Read the model definition and answer for the solid it produces. Units are mm, in the model's axes. A direction names the side the tool comes from. Coordinates: 2 decimals unless noted, no trailing zeros. Write each loop counter-clockwise with the first axis right and the second up, starting at its lowest first coordinate (ties: lowest second). Pieces come first, ordered by that corner, then holes. Notation, with made-up numbers: (34, 58.25) - (49, 58.25) arc R31 cw to (49, 82.25) - close; hole circle Ø10 at (47.25, -39). An arc over 180 degrees is marked (long way). Return JSON: item names as keys, results as strings.
```python
from build123d import *

# Parameters (mm, degrees)
F1_DEPTH = 500
F2_DEPTH = 311.15


with BuildPart() as f1:
    # F0 (on Front) → F1 (new body)
    with BuildSketch(Plane.XZ):
        with BuildLine():
            ThreePointArc((-155.575, 0), (0, -155.575), (155.575, 0))
            ThreePointArc((155.575, 0), (0, 155.575), (-155.575, 0))
        make_face()
    extrude(amount=F1_DEPTH)

    # F0 (on Front) → F2 (join)
    with BuildSketch(Plane.XZ):
        with BuildLine():
            ThreePointArc((-155.575, 0), (0, -155.575), (155.575, 0))
            ThreePointArc((155.575, 0), (0, 155.575), (-155.575, 0))
        make_face()
        with BuildLine():
            Line((155.575, -200), (155.575, 0))
            ThreePointArc((155.575, 0), (0, -155.575), (-155.575, 0))
            Line((-155.575, 0), (-155.575, -200))
            Line((-155.575, -200), (155.575, -200))
        make_face()
    extrude(amount=-F2_DEPTH)


solid = f1.part
```
(1) Straight lines are drawn through the part: line 1 (Z direction, x = -5, y = -41.5); line 2 (Z direction, x = 71.5, y = -146); line 3 (X direction, y = -204, z = 140.5). For each, find the intervals that lie inside material, in ascending order. Write a range as from..to.
Answer:
{"line 1": "-155.49..155.49", "line 2": "-138.17..138.17", "line 3": "-66.81..66.81"}
(2) Flat-ended cylindrical pins translate along their axes: P1, Ø1.5, axis at y = -179.5, z = 79.5, coming from the +X side; P2, Ø1.5, axis at y = -87, z = -89, coming from the +X side; P3, Ø10, axis at y = -241, z = 113.5, coming from the -X side. Find the tip coordinate at first contact, or state that the pin passes through.
Answer:
{"P1": "x = 134.17", "P2": "x = 128.12", "P3": "x = -111.5"}
(3) A cutting plane is placed at D-D (x = 0). Determine the outline of the cut face in (y, z) (3 decimals), and give its area (3 significant figures).
Answer:
{"outline": "(-500, -155.575) - (0, -155.575) - (0, -200) - (311.15, -200) - (311.15, 155.575) - (-500, 155.575) - close", "area": "266,000 mm²"}
(4) Which of the six approach directions +Z, -Z, +X, -X, +Y, -Y give full straight-line access (tool end or side, diameter ignored) to faces 1 (the face through (-2, 0, -165)), 2 (the face through (155.575, 153, -101))?
Answer:
{"face 1": "-Z, -Y", "face 2": "+Z, -Z, +X, +Y, -Y"}
(5) A cutting plane is placed at C-C (y = 184). Determine the outline of the cut face in (x, z) (3 decimals).
Answer:
{"outline": "(-155.575, -200) - (155.575, -200) - (155.575, 0) arc R155.575 ccw to (-155.575, 0) - close"}
(6) A cutting plane is placed at B-B (x = -124). Determine the outline of the cut face in (y, z), and give its area (3 significant figures).
Answer:
{"outline": "(-500, -93.96) - (0, -93.96) - (0, -200) - (311.15, -200) - (311.15, 93.96) - (-500, 93.96) - close", "area": "185,000 mm²"}
(7) A cutting plane is placed at A-A (z = -45.5). Determine the outline of the cut face in (x, y) (3 decimals).
Answer:
{"outline": "(-155.575, 0) - (-148.773, 0) - (-148.773, -500) - (148.773, -500) - (148.773, 0) - (155.575, 0) - (155.575, 311.15) - (-155.575, 311.15) - close"}
